Autodesk Fusion 360 part; units mm, degrees
sketch "Sketch1" plane through (0, 0, 0) normal (0, 0, 1) x (1, 0, 0)
  circle A0 centre (7.5, 10) radius 1.8
  line L0 (0, 0) -> (15, 0)
  line L1 (15, 0) -> (15, 20)
  line L2 (15, 20) -> (0, 20)
  line L3 (0, 20) -> (0, 0)
  circle A1 centre (7.5, 10) radius 3.5
  line L4 (15, 20) -> (0, 20)
  line L5 (0, 20) -> (0, 28)
  line L6 (0, 28) -> (15, 28)
  line L7 (15, 28) -> (15, 20)
  dimension "d3" = 3.6
  dimension "d17" = 15
  dimension "d18" = 20
  dimension "d19" = 10
  dimension "d21" = 7
  dimension "d26" = 15
  dimension "d27" = 8
extrude "Extrude1" add sketch "Sketch1" along normal blind 7 contours L0 L1 L2 L3 L4 | A1
sketch "Sketch4" plane through (15, 0, 0) normal (1, 0, 0) x (0, 1, 0)
  line L0 (0, 0) -> (20, 0)
  line L1 (20, 0) -> (20, 7)
  line L2 (20, 7) -> (0, 7)
  line L3 (0, 7) -> (0, 0)
extrude "Extrude4" cut sketch "Sketch1" along normal blind 4 contours A1
extrude "Extrude5" add sketch "Sketch1" along normal blind 26 contours L2 L4 L5 L6 L7
extrude "Extrude6" add sketch "Sketch4" along normal blind 35
sketch "Sketch5" plane through (0, 0, 0) normal (0, 0, -1) x (1, 0, 0)
  circle A0 centre (7.5, -10) radius 3.5
  line L0 (50, 0) -> (0, 0)
  line L1 (0, 0) -> (0, -28)
  line L2 (0, -28) -> (15, -28)
  line L3 (15, -28) -> (15, -20)
  line L4 (15, -20) -> (50, -20)
  line L5 (50, -20) -> (50, 0)
  circle A1 centre (42.5, -10) radius 1.8
  circle A2 centre (42.5, -10) radius 3.5
  circle A3 centre (30.5, -10) radius 1.8
  circle A4 centre (30.5, -10) radius 3.5
  point P0 (7.5, -10)
  dimension "d33" = 3.6
  dimension "d34" = 7
  dimension "d35" = 7.5
  dimension "d40" = 3.6
  dimension "d41" = 7
  dimension "d42" = 12
extrude "Extrude8" cut sketch "Sketch5" against normal through all contours A1 | A3
extrude "Extrude7" cut sketch "Sketch5" against normal blind 5 contours A1 | A2 | A4
chamfer "Chamfer2" distance 1 angle 45 2 faces at (7.4128, 20.4967, 0) (5, 28, 8.6667)
equation "d19 = d18 / 2"
equation "d33 = d3"
equation "d34 = d21"
equation "d36 = -d7 + 2 mm"
equation "d40 = d3"
equation "d41 = d21"
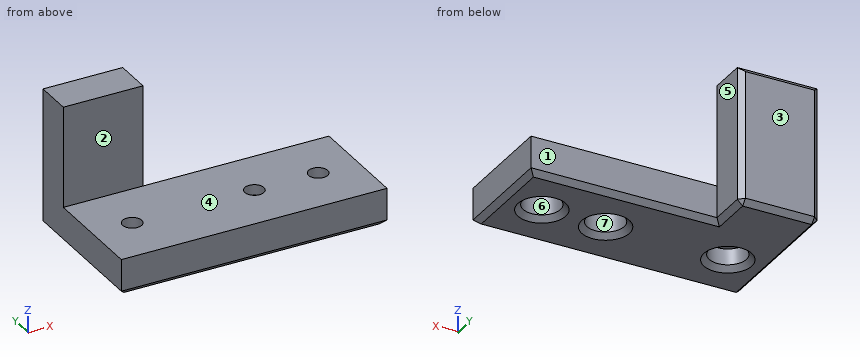
Geometry check sheet. Reference: the model listing, model coordinates, mm. Face numbers are marked on the shaded views. A direction names the side the tool comes from. Coordinates: 2 decimals unless noted, no trailing zeros. Order: outer loops, then holes, each group sorted by start corner. A loop starts at its lowest first (then second) coordinate and runs counter-clockwise, first axis right, second up. Notation, with made-up numbers: (-17.5, -10.5) -> (38.5, -10.5) arc R31 ccw to (38.5, 28.5) -> close; hole circle Ø10 at (78.5, -1). An arc over 180 degrees is marked (long way). Use a Markdown table: item, result. Add a question column.
1. Go/stop test with flat-tipped pins: pin 1 Ø4 at (x, y) = (7.5, 10) entering from +Z; pin 2 Ø2 at (x, y) = (7.5, 9.5) entering from -Z; pin 3 Ø8 at (x, y) = (7.5, 10) entering from -Z; pin 4 Ø1 at (y, z) = (21.5, 14) entering from +X. Record where each tip stops, or that it passes through.
2. Cross-section at A-A (x = 42.5). Enter the section's corners in (y, z).
3. Cross-section at B-B (z = 3). Enter the section's corners in (x, y), and give its area (3 significant figures).
4. Material ranges on L1, parallel to Y at x = 7.5, z = 2.65; L2, parallel to Y at x = 42.5, z = 6.55; L3, parallel to X at y = 10.5, z = 4.5, recorded low to high.
5. Cross-section at D-D (y = 2.75). Enter the section's corners in (x, z), and give its area (3 significant figures).
6. Cross-section at C-C (x = 7.5). Enter the section's corners in (y, z), and give its area (3 significant figures).
7. Set-up check for the marked faces 1, 2 and 3: record each of +Z, -Z, +X, -X, +Y, -Y from which the full face is reachable in a straight line by a thin tool's end or side.
8. Mould release check, pull along X, two halves, no side actions. Record for the marked faces 4, 5, 6 and 7: pulls with the +X half, pulls with the -X half, needs draft (parallel to the pull), parting line crosses it, or undercut.
Filled sheet:
| question | item | result |
|---|---|---|
| 1 | pin 1 | z = 7 |
| 1 | pin 2 | through |
| 1 | pin 3 | z = 0.5 |
| 1 | pin 4 | x = 15 |
| 2 | outline | (0, 1) -> (1, 0) -> (5.5, 0) -> (6.5, 1) -> (6.5, 5) -> (8.2, 5) -> (8.2, 7) -> (0, 7) -> close; (11.8, 5) -> (13.5, 5) -> (13.5, 1) -> (14.5, 0) -> (19, 0) -> (20, 1) -> (20, 7) -> (11.8, 7) -> close |
| 3 | outline | (0, 0) -> (50, 0) -> (50, 20) -> (15, 20) -> (15, 27) -> (14, 28) -> (1, 28) -> (0, 27) -> close; hole circle Ø7 at (7.5, 10); hole circle Ø7 at (30.5, 10); hole circle Ø7 at (42.5, 10) |
| 3 | area | 1,000 mm2 |
| 4 | L1 | 0 to 6.5, 13.5 to 28 |
| 4 | L2 | 0 to 8.2, 11.8 to 20 |
| 4 | L3 | 0 to 5.77, 9.23 to 27.04, 33.96 to 39.04, 45.96 to 50 |
| 5 | outline | (0, 1) -> (1, 0) -> (49, 0) -> (50, 1) -> (50, 7) -> (0, 7) -> close |
| 5 | area | 349 mm2 |
| 6 | outline | (0, 1) -> (1, 0) -> (5.5, 0) -> (6.5, 1) -> (6.5, 4) -> (8.2, 4) -> (8.2, 7) -> (0, 7) -> close; (11.8, 4) -> (13.5, 4) -> (13.5, 1) -> (14.5, 0) -> (27, 0) -> (28, 1) -> (28, 25) -> (27, 26) -> (20, 26) -> (20, 7) -> (11.8, 7) -> close |
| 6 | area | 307 mm2 |
| 7 | face 1 | +Z, -Z, +X, +Y |
| 7 | face 2 | +Z, +X, -X, -Y |
| 7 | face 3 | +Z, -Z, +X, -X, +Y |
| 8 | face 4 | needs draft |
| 8 | face 5 | pulls with the +X half |
| 8 | face 6 | undercut |
| 8 | face 7 | undercut |
